Autodesk Inventor part; units mm, degrees
ref_plane "YZ Plane" through (0, 0, 0) normal (1, 0, 0) x (0, 1, 0)
ref_plane "XZ Plane" through (0, 0, 0) normal (0, 1, 0) x (-1, 0, 0)
ref_plane "XY Plane" through (0, 0, 0) normal (0, 0, 1) x (1, 0, 0)
sketch "Sketch1" plane through (0, 0, 0) normal (1, 0, 0) x (0, 1, 0)
  circle A0 centre (0, 0) radius 20
  dimension "d0" = 40
extrude "Extrusion1" add sketch "Sketch1" along normal blind 5
sketch "Sketch2" plane through (5, 0, 0) normal (1, 0, 0) x (0, 0, -1)
  circle A0 centre (0, 0) radius 21
  dimension "d3" = 42
extrude "Extrusion2" add sketch "Sketch2" along normal mid plane 2
sketch "Sketch3" plane through (0, 0, 0) normal (-1, 0, 0) x (0, 0, 1)
  circle A0 centre (0, 0) radius 21
extrude "Extrusion3" add sketch "Sketch3" against normal blind 2
fillet "Fillet1" radius 0.5 2 edges at (2, -20, 0) (4, -20, 0)
sketch "Sketch4" plane through (6, 0, 0) normal (1, 0, 0) x (0, 0, -1)
  circle A0 centre (0, 0) radius 18.5
  dimension "d9" = 37
extrude "Extrusion4" cut sketch "Sketch4" against normal blind 6
sketch "Sketch5" plane through (6, 0, 0) normal (1, 0, 0) x (0, 0, -1)
  circle A0 centre (0, 0) radius 2
  circle A1 centre (0, 0) radius 3
  dimension "d12" = 4
  dimension "d13" = 6
extrude "Extrusion5" add sketch "Sketch5" against normal blind 6
sketch "Sketch6" plane through (6, 0, 0) normal (1, 0, 0) x (0, 0, -1)
  point P0 (0, 0)
sketch "Sketch7" plane through (6, 0, 0) normal (1, 0, 0) x (0, 0, -1)
  circle A0 centre (0, 0) radius 3
  circle A1 centre (0, 0) radius 24.6795
sketch "Sketch8" plane through (0, 0, 0) normal (-1, 0, 0) x (0, 0, 1)
  circle A0 centre (0, 0) radius 27.0731
extrude "Extrusion6" cut sketch "Sketch8" against normal blind 1
extrude "Extrusion7" cut sketch "Sketch7" against normal blind 1
sketch "Sketch9" plane through (6, 0, 0) normal (1, 0, 0) x (0, 0, -1)
  circle A0 centre (0, 0) radius 11.2863
extrude "Extrusion8" cut sketch "Sketch9" against normal blind 1
sketch "Sketch10" plane through (5, 0, 0) normal (1, 0, 0) x (0, 0, -1)
  line L0 (-2.72, 0) -> (-2.72, 1) construction
  line L1 (-2.72, 1) -> (-2.72, -1) construction
  line L2 (-2.72, 1) -> (-19.124, 1)
  line L3 (-19.124, 1) -> (-19.124, -1)
  line L4 (-19.124, -1) -> (-2.72, -1)
  line L5 (-2.72, -1) -> (-2.72, 1)
  point P0 (0, 0)
  dimension "d22" = 1
  dimension "d23" = 2
  dimension "d24" = 2
extrude "Extrusion9" add sketch "Sketch10" against normal blind 4
pattern_circular "Circular Pattern1" count 4 over 360 about axis through (6, 0, 0) along (-1, 0, 0) of "Extrusion9"
sketch "Sketch11" plane through (1, 0, 0) normal (-1, 0, 0) x (0, 0, 1)
  circle A0 centre (0, 0) radius 2
  circle A1 centre (0, 0) radius 1.5
  dimension "d30" = 3
extrude "Extrusion10" add sketch "Sketch11" against normal blind 4
properties part number "mtv_brakeWheel_1-13"
Check sheet for the modelled part. Datum: model origin and axes. Units: mm. A direction names the side the tool comes from. Round coordinates to 2 decimals unless told otherwise and drop trailing zeros. Loops run counter-clockwise (first coordinate to the right, second up) from the corner with the lowest first, then second, coordinate; pieces in that order, holes last. Notation, with made-up numbers: (76, 24) - (111, 24) arc R15 cw to (111, 29) - close; hole circle Ø10 at (-27.5, -33). An arc over 180 degrees is marked (long way). Answer as a JSON object with one key per item and string values. Group by question number.
Q1. Scan lines: line 1 along Y through (x, z) = (1.95, 0); line 2 along Z through (x, y) = (1.55, 10.5); line 3 along Y through (x, z) = (2.45, 0). Record each from-to range of solid material in increasing order. Write a range as [from, to].
Q2. Mould release check, pull along X, two halves, no side actions. Record for faces 4 (the face through (1, 0, 4)), 5 (the face through (2, -9.2, 18.6)), 6 (the face through (2.97, 0.07, -1.5)): released by +X, released by -X, zero draft, split by the parting line, or undercut.
Q3. Set-up check for faces 1 (the face through (3.03, -2.13, -2.11)), 2 (the face through (5, 0, 4)), 3 (the face through (2.993, -4.336, 19.524)): record each of +Z, -Z, +X, -X, +Y, -Y from which the full face is reachable in a straight line by a thin tool's end or side.
Q4. Gauge pin test, flat ends, axial feed: P1, Ø1.2, axis at x = 3, y = -14.5, coming from the +Z side; P2, Ø2, axis at x = 3.5, y = -9.5, coming from the -Z side; P3, Ø2, axis at x = 2.5, z = 8, coming from the +Y side. Record the tip position at first contact, or that the pin passes through.
Q5. Sectioned sample at A-A, the plane y = 0. Enter the section's corners in (x, z), plus the area to 3 significant figures.
Q6. Sectioned sample at C-C, the plane y = 7. Count the separate pieces of the cut face and the enclosed holes in it, plus the area to 3 significant figures.
Solution:
{
 "1": {"line 1": "y = [-21, -1.5], [1.5, 21]", "line 2": "z = [-18.19, -15.23], [-1, 1], [15.23, 18.19]", "line 3": "y = [-20, -1.5], [1.5, 20]"},
 "2": {"face 4": "released by -X", "face 5": "undercut", "face 6": "zero draft"},
 "3": {"face 1": "+X, -X", "face 2": "+Z, -Z, +X, +Y, -Y", "face 3": "none"},
 "4": {"P1": "stops at z = 14.38", "P2": "stops at z = -19.14", "P3": "stops at y = 19.75"},
 "5": {"outline": "(1, -21) - (2, -21) - (2, -20.5) arc R0.5 cw to (2.5, -20) - (3.5, -20) arc R0.5 cw to (4, -20.5) - (4, -21) - (5, -21) - (5, -1.5) - (1, -1.5) - close; (1, 1.5) - (5, 1.5) - (5, 21) - (4, 21) - (4, 20.5) arc R0.5 cw to (3.5, 20) - (2.5, 20) arc R0.5 cw to (2, 20.5) - (2, 21) - (1, 21) - close", "area": "152 mm²"},
 "6": {"separate pieces": "3", "enclosed holes": "0", "area": "25.4 mm²"}
}
